For this review, use the dimensioned drawing (mm, ordinates from the lowest corner) and the shaded views. A direction names the side the tool comes from. Give positions to 0.01 mm unless a question says otherwise; leave off trailing zeros. Write each loop counter-clockwise with the first axis right and the second up, starting at its lowest first coordinate (ties: lowest second). Pieces come first, ordered by that corner, then holes. Notation, with made-up numbers: M 79,84.5 L 86,84.5 A22 cw 86,101.5 Z; hole C 73.25,-12.75 d5. An arc over 180 degrees is marked long. Write each question's results on one line, items separated by ' | '. Start each with the question number.
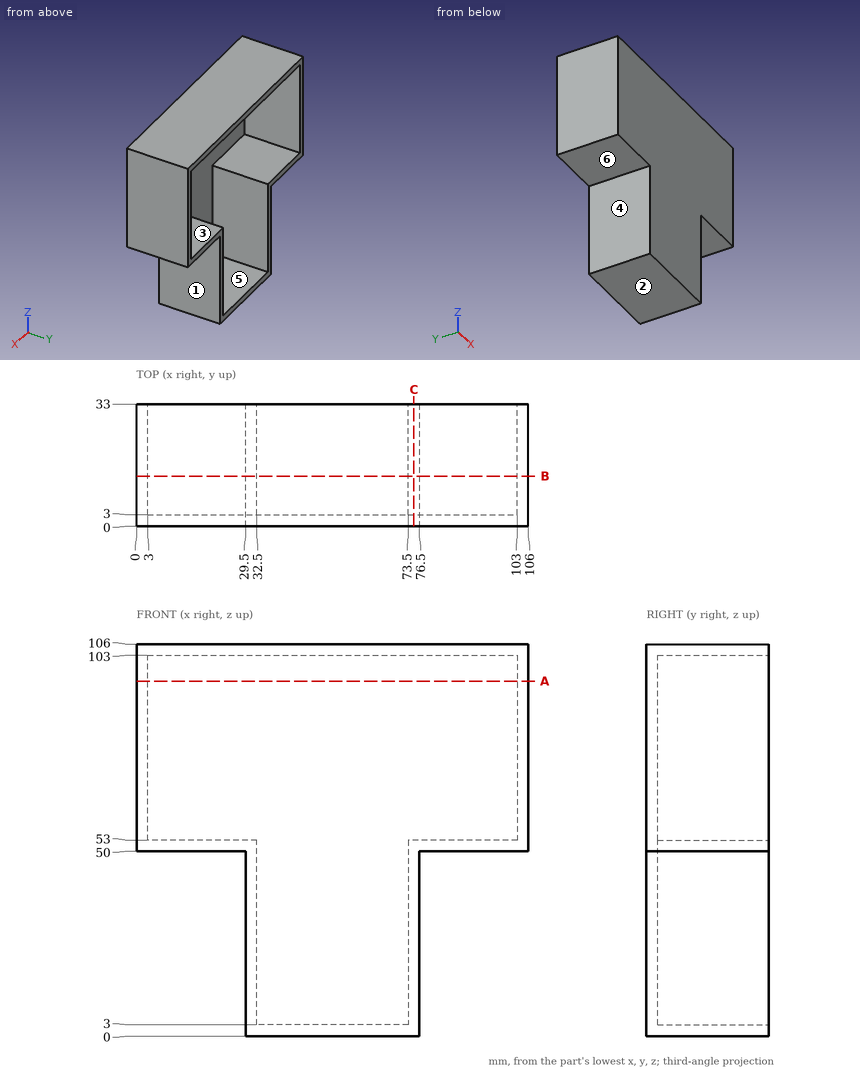
(1) Add section C-C (x = 75). State the section outline as (y, z) points, then the cut area to 3 significant figures.
(2) Wall thickness on L1, parallel to Z at x = 38, y = 7; L2, parallel to Z at x = 22.5, y = 21: over which ranges is each line inside the solid? List them lowest first.
(3) Machinability: for the marked faces 1, 2 and 3, which of the approach directions +Z, -Z, +X, -X, +Y, -Y give a long, thin tool a straight path to every point of the face, cutting with its end or side? Answer none if there is none.
(4) Draft analysis for pull direction Z (two halves, no side actions). For the marked faces 4, 5 and 6, state which applies: pulls with the +Z half, pulls with the -Z half, needs draft (parallel to the pull), parting line crosses it, or undercut.
(5) Clearance check with flat-ended pins moving along their axes: P1, Ø15, axis at y = 25, z = 34.5, coming from the +X side; P2, Ø4, axis at x = 80.5, z = 58.5, coming from the +Y side; P3, Ø9, axis at x = 18.5, y = 20, coming from the -Z side. State where each tip first meets the part, or that it passes through.
(6) Add section A-A (z = 96). State the section outline as (x, y) points.
(7) Add section B-B (y = 13.5). State the section outline as (x, z) points.
Calculated:
1) outline: M 0,0 L 33,0 L 33,53 L 3,53 L 3,103 L 33,103 L 33,106 L 0,106 Z | area: 2,000 mm²
2) L1: z = 0 to 3, 103 to 106 | L2: z = 50 to 53, 103 to 106
3) face 1: -Z, +X, +Y, -Y | face 2: -Z, +X, -X, +Y, -Y | face 3: +Y
4) face 4: needs draft | face 5: undercut | face 6: pulls with the -Z half
5) P1: stops at x = 76.5 | P2: stops at y = 3 | P3: stops at z = 50
6) outline: M 0,0 L 106,0 L 106,33 L 103,33 L 103,3 L 3,3 L 3,33 L 0,33 Z
7) outline: M 0,50 L 29.5,50 L 29.5,0 L 76.5,0 L 76.5,50 L 106,50 L 106,106 L 0,106 Z; hole M 3,53 L 32.5,53 L 32.5,3 L 73.5,3 L 73.5,53 L 103,53 L 103,103 L 3,103 Z
